```python
from build123d import *

# Parameters (mm, degrees)
SKETCH_1_W      = 195
SKETCH_1_H      = 170
SKETCH_1_R      = 5
EXTRUDE_1_DEPTH = 100
CHAMFER_1_SIZE  = 10


with BuildPart() as part:
    # 草图1 → 凸台-拉伸1 (new body)
    with BuildSketch(Plane.XY):
        with Locations((40, 0)):
            Rectangle(SKETCH_1_W, SKETCH_1_H)
        with Locations((-37.5, 65)):
            Circle(SKETCH_1_R, mode=Mode.SUBTRACT)
        with Locations((37.5, 65)):
            Circle(SKETCH_1_R, mode=Mode.SUBTRACT)
        with Locations((-37.5, -65)):
            Circle(SKETCH_1_R, mode=Mode.SUBTRACT)
        with Locations((37.5, -65)):
            Circle(SKETCH_1_R, mode=Mode.SUBTRACT)
    extrude(amount=EXTRUDE_1_DEPTH)

    # 倒角1
    chamfer_1_edges = [part.edges().sort_by_distance(p)[0] for p in [
        (137.5, -85, 50),
        (-57.5, -85, 50),
        (-57.5, 85, 50),
        (137.5, 85, 50),
    ]]
    chamfer(chamfer_1_edges, length=CHAMFER_1_SIZE)


solid = part.part
```
Build history of the part. All positions in model axes, mm. Round coordinates to 2 decimals unless told otherwise and drop trailing zeros. Write each loop counter-clockwise with the first axis right and the second up, starting at its lowest first coordinate (ties: lowest second). Pieces come first, ordered by that corner, then holes. Notation, with made-up numbers: (80.5, 14.25) - (88.5, 14.25) arc R18 cw to (88.5, 28.25) - close; hole circle Ø3 at (-29.75, 54). An arc over 180 degrees is marked (long way). Write each question's results on one line, items separated by ' | '. Start each with the question number.
Item 1: Mould opens along Y. For faces 1 (the face through (-52.4, -80.1, 49.3)), 2 (the face through (-52.4, 80.1, 49.3)), 3 (the face through (33.815, 68.379, 49.3)) say: pulls with the +Y half, pulls with the -Y half, needs draft (parallel to the pull), parting line crosses it, or undercut.
Item 2: Drop a flat-ended pin along its axis: P1, Ø6, axis at x = 37.5, y = 65, coming from the -Z side. Give the stop position or say it passes through.
Item 3: Saw through at C-C (x = -37.5). Write the cut outline in (y, z), and give its area (3 significant figures).
Item 4: Saw through at A-A (z = 12). Write the cut outline in (x, y), and give its area (3 significant figures).
Item 5: Saw through at B-B (y = -65). Write the cut outline in (x, z), and give its area (3 significant figures).
Item 6: Wall check: L1, parallel to Y at x = -37.5, z = 39; L2, parallel to Y at x = -38.5, z = 27; L3, parallel to X at y = 67, z = 93. Give the ranges that are in metal, low to high. Write a range as [from, to].
Results are:
1) face 1: pulls with the -Y half | face 2: pulls with the +Y half | face 3: undercut
2) P1: passes through
3) outline: (-85, 0) - (-70, 0) - (-70, 100) - (-85, 100) - close; (-60, 0) - (60, 0) - (60, 100) - (-60, 100) - close; (70, 0) - (85, 0) - (85, 100) - (70, 100) - close | area: 15,000 mm²
4) outline: (-57.5, -75) - (-47.5, -85) - (127.5, -85) - (137.5, -75) - (137.5, 75) - (127.5, 85) - (-47.5, 85) - (-57.5, 75) - close; hole circle Ø10 at (-37.5, -65); hole circle Ø10 at (-37.5, 65); hole circle Ø10 at (37.5, -65); hole circle Ø10 at (37.5, 65) | area: 32,600 mm²
5) outline: (-57.5, 0) - (-42.5, 0) - (-42.5, 100) - (-57.5, 100) - close; (-32.5, 0) - (32.5, 0) - (32.5, 100) - (-32.5, 100) - close; (42.5, 0) - (137.5, 0) - (137.5, 100) - (42.5, 100) - close | area: 17,500 mm²
6) L1: y = [-85, -70], [-60, 60], [70, 85] | L2: y = [-85, -69.9], [-60.1, 60.1], [69.9, 85] | L3: x = [-57.5, -42.08], [-32.92, 32.92], [42.08, 137.5]
